Source: three-view drawing plus pictorial views. Frame: mm from the lowest corner of the part. A direction names the side the tool comes from. Give positions to 0.01 mm unless a question says otherwise; leave off trailing zeros. Order: outer loops, then holes, each group sorted by start corner. A loop starts at its lowest first (then second) coordinate and runs counter-clockwise, first axis right, second up.
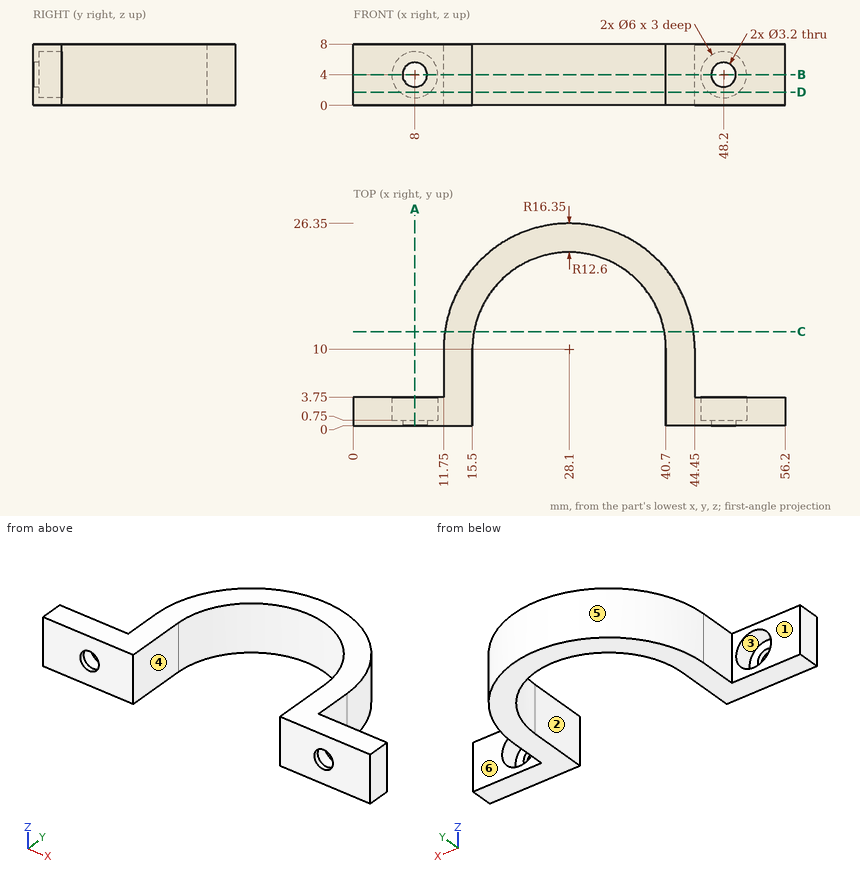
(1) Access query for the marked faces 1, 2 and 3. Directions: +Z, -Z, +X, -X, +Y, -Y. A direction counts if a zero-diameter tool reaches every point of the face in a straight line with its end or side. Return the directions, or none.
(2) Section C-C, the plane y = 12.25. Return loops of the section in (x, z) (1 decimal).
(3) Draft query along X for the marked faces 4, 5 and 6. Return one class per face: +X half, -X half, draft (parallel to the pull), parting line (faces both ways), or undercut.
(4) Section A-A, the plane x = 8. Return loops of the section in (y, z).
(5) Pin query (flat end, axial travel): pin 1 Ø4 at (x, z) = (23, 5) entering from -Y; pin 2 Ø4 at (x, z) = (4, 4) entering from +Y; pin 3 Ø1.9 at (y, z) = (5.5, 5.5) entering from -X. Return the tip coordinate at first contact, or that it passes through.
(6) Section B-B, the plane z = 4. Return loops of the section in (x, y).
(7) Section D-D, the plane z = 1.75. Return loops of the section in (x, y).
(8) Line query: line 1 along X through (y, z) = (0.4, 4); line 2 along X through (y, z) = (2.45, 4); line 3 along X through (y, z) = (8.5, 6.25). Output: solid intervals per line, ascending.
Checks:
1. face 1: +Z, -Z, -X, +Y
1. face 2: +Z, -Z, -Y
1. face 3: +Y
2. outline: (11.9, 0) - (15.7, 0) - (15.7, 8) - (11.9, 8) - close; (40.5, 0) - (44.3, 0) - (44.3, 8) - (40.5, 8) - close
3. face 4: undercut
3. face 5: parting line
3. face 6: draft
4. outline: (0, 0) - (3.75, 0) - (3.75, 1) - (0.75, 1) - (0.75, 2.4) - (0, 2.4) - close; (0, 5.6) - (0.75, 5.6) - (0.75, 7) - (3.75, 7) - (3.75, 8) - (0, 8) - close
5. pin 1: stops at y = 20.41
5. pin 2: stops at y = 3.75
5. pin 3: stops at x = 11.75
6. outline: (0, 0) - (6.4, 0) - (6.4, 0.75) - (5, 0.75) - (5, 3.75) - (0, 3.75) - close; (9.6, 0) - (15.5, 0) - (15.5, 10.1) arc R12.6 cw to (40.7, 10.1) - (40.7, 0) - (46.6, 0) - (46.6, 0.75) - (45.2, 0.75) - (45.2, 3.75) - (44.45, 3.75) - (44.45, 10.1) arc R16.35 ccw to (11.75, 10.1) - (11.75, 3.75) - (11, 3.75) - (11, 0.75) - (9.6, 0.75) - close; (49.8, 0) - (56.2, 0) - (56.2, 3.75) - (51.2, 3.75) - (51.2, 0.75) - (49.8, 0.75) - close
7. outline: (0, 0) - (15.5, 0) - (15.5, 10.1) arc R12.6 cw to (40.7, 10.1) - (40.7, 0) - (56.2, 0) - (56.2, 3.75) - (50.18, 3.75) - (50.18, 0.75) - (46.22, 0.75) - (46.22, 3.75) - (44.45, 3.75) - (44.45, 10.1) arc R16.35 ccw to (11.75, 10.1) - (11.75, 3.75) - (9.98, 3.75) - (9.98, 0.75) - (6.02, 0.75) - (6.02, 3.75) - (0, 3.75) - close
8. line 1: x = 0 to 6.4, 9.6 to 15.5, 40.7 to 46.6, 49.8 to 56.2
8. line 2: x = 0 to 5, 11 to 15.5, 40.7 to 45.2, 51.2 to 56.2
8. line 3: x = 11.75 to 15.5, 40.7 to 44.45
